Source: CAD feature listing. Evaluate the final solid. Frame: model axes, mm. A direction names the side the tool comes from. Give positions to 0.01 mm unless a question says otherwise; leave off trailing zeros. Write each loop counter-clockwise with the first axis right and the second up, starting at its lowest first coordinate (ties: lowest second). Pieces come first, ordered by that corner, then holes. Notation, with made-up numbers: (22, -36) -> (59, -36) arc R10 cw to (59, -29) -> close; hole circle Ø8 at (16, 28). An arc over 180 degrees is marked (long way). Answer as a JSON object with one key per item and string values. Group by question number.
Item 1: Section query D-D on x = 7.5. Return the cut outline in (y, z), plus the area to 3 significant figures.
Item 2: Ray query, probe 1 along Y at (x, z) = (15, 0.8); probe 2 along X at (y, z) = (-6, 2.1); probe 3 along Z at (x, y) = (8, -1). Return the intervals inside material, ascending. Write a range as from..to.
Item 3: Access query for faces 1 (the face through (-8, -2.465, 2)), 2 (the face through (-4.62, 8.66, 2.39)), 3 (the face through (-8, -8.965, 2)), 4 (the face through (-4.339, 6, 2)), 5 (the face through (-4.64, 2.75, 2.39)). Directions: +Z, -Z, +X, -X, +Y, -Y. A direction counts if a zero-diameter tool reaches every point of the face in a straight line with its end or side. Return the directions, or none.
Item 4: Section query A-A on z = 2.6. Return the cut outline in (x, y), plus the area to 3 significant figures.
Item 5: First-contact query: pin 1 Ø1.8 at (y, z) = (6.5, 3) entering from -X; pin 2 Ø1.8 at (y, z) = (-5.5, 2.5) entering from +X; pin 3 Ø11 at (x, y) = (4, 0.5) entering from +Z. Flat tips, straight axial feed; report the tip coordinate or a pass-through.
Item 6: Pull-direction query (X, two-part tool) for faces 6 (the face through (0, 18.05, 1)), 7 (the face through (-10.839, -6, 2)), 8 (the face through (-16.5, 15.07, 0.6)); classes: pulls with the +X half, pulls with the -X half, needs draft (parallel to the pull), parting line crosses it, or undercut.
Item 7: Section query B-B on x = -15. Return the cut outline in (y, z).
from build123d import *

# Parameters (mm, degrees)
F0_W     = 36.1
F0_H     = 36.1
F0_R     = 1.5
F1_DEPTH = 1.22
F2_R     = 2.5
F3_W     = 6.5
F3_H     = 6.5
F4_DEPTH = 2.3
F5_R     = 1


with BuildPart() as f1:
    # F0 (on Top) → F1 (new body)
    with BuildSketch(Plane.XY):
        Rectangle(F0_W, F0_H)
        with Locations((-15, -15)):
            Circle(F0_R, mode=Mode.SUBTRACT)
        with Locations((15, -15)):
            Circle(F0_R, mode=Mode.SUBTRACT)
        with Locations((-15, 15)):
            Circle(F0_R, mode=Mode.SUBTRACT)
        with Locations((15, 15)):
            Circle(F0_R, mode=Mode.SUBTRACT)
    extrude(amount=F1_DEPTH)

    # F2
    f2_edges = [f1.edges().sort_by_distance(p)[0] for p in [
        (18.05, 18.05, 0.61),
        (18.05, -18.05, 0.61),
        (-18.05, -18.05, 0.61),
        (-18.05, 18.05, 0.61),
    ]]
    fillet(f2_edges, radius=F2_R)

    # F3 (on face) → F4 (join)
    with BuildSketch(Plane.XY.offset(1.22)):
        with Locations((-7.588814, -5.71497)):
            Rectangle(F3_W, F3_H)
        with Locations((-7.588814, 5.71497)):
            Rectangle(F3_W, F3_H)
    extrude(amount=F4_DEPTH)

    # F5
    f5_edges = [f1.edges().sort_by_distance(p)[0] for p in [
        (-10.838814, -8.96497, 2.37),
        (-4.338814, -8.96497, 2.37),
        (-4.338814, -2.46497, 2.37),
        (-10.838814, -2.46497, 2.37),
        (-10.838814, 8.96497, 2.37),
        (-10.838814, 2.46497, 2.37),
        (-4.338814, 8.96497, 2.37),
        (-4.338814, 2.46497, 2.37),
    ]]
    fillet(f5_edges, radius=F5_R)


solid = f1.part
Worked answers:
{
 "1": {"outline": "(-18.05, 0) -> (18.05, 0) -> (18.05, 1.22) -> (-18.05, 1.22) -> close", "area": "44.0 mm^2"},
 "2": {"probe 1": "-18.05..-16.5, -13.5..13.5, 16.5..18.05", "probe 2": "-10.84..-4.34", "probe 3": "0..1.22"},
 "3": {"face 1": "+Z, +X, -X", "face 2": "+Z, +X, +Y", "face 3": "+Z, +X, -X, -Y", "face 4": "+Z, +X, +Y, -Y", "face 5": "+Z, +X"},
 "4": {"outline": "(-10.84, -7.96) arc R1 ccw to (-9.84, -8.96) -> (-5.34, -8.96) arc R1 ccw to (-4.34, -7.96) -> (-4.34, -3.46) arc R1 ccw to (-5.34, -2.46) -> (-9.84, -2.46) arc R1 ccw to (-10.84, -3.46) -> close; (-10.84, 3.46) arc R1 ccw to (-9.84, 2.46) -> (-5.34, 2.46) arc R1 ccw to (-4.34, 3.46) -> (-4.34, 7.96) arc R1 ccw to (-5.34, 8.96) -> (-9.84, 8.96) arc R1 ccw to (-10.84, 7.96) -> close", "area": "82.8 mm^2"},
 "5": {"pin 1": "x = -10.84", "pin 2": "x = -4.34", "pin 3": "z = 1.22"},
 "6": {"face 6": "needs draft", "face 7": "pulls with the -X half", "face 8": "undercut"},
 "7": {"outline": "(-18.05, 0) -> (-16.5, 0) -> (-16.5, 1.22) -> (-18.05, 1.22) -> close; (-13.5, 0) -> (13.5, 0) -> (13.5, 1.22) -> (-13.5, 1.22) -> close; (16.5, 0) -> (18.05, 0) -> (18.05, 1.22) -> (16.5, 1.22) -> close"}
}
